Geometry: see drawing. Coordinates: mm, zero at the bounding-box minimum. Round coordinates to 2 decimals unless told otherwise and drop trailing zeros. Write each loop counter-clockwise with the first axis right and the second up, starting at its lowest first coordinate (ties: lowest second). Pieces come first, ordered by that corner, then holes. Notation, with made-up numbers: (7.5, 37.5) - (11.5, 37.5) arc R17 ccw to (11.5, 56.5) - close; hole circle Ø1 at (77, 76.25). An arc over 180 degrees is marked (long way). One line per item, written item: value. Start each with the question number.
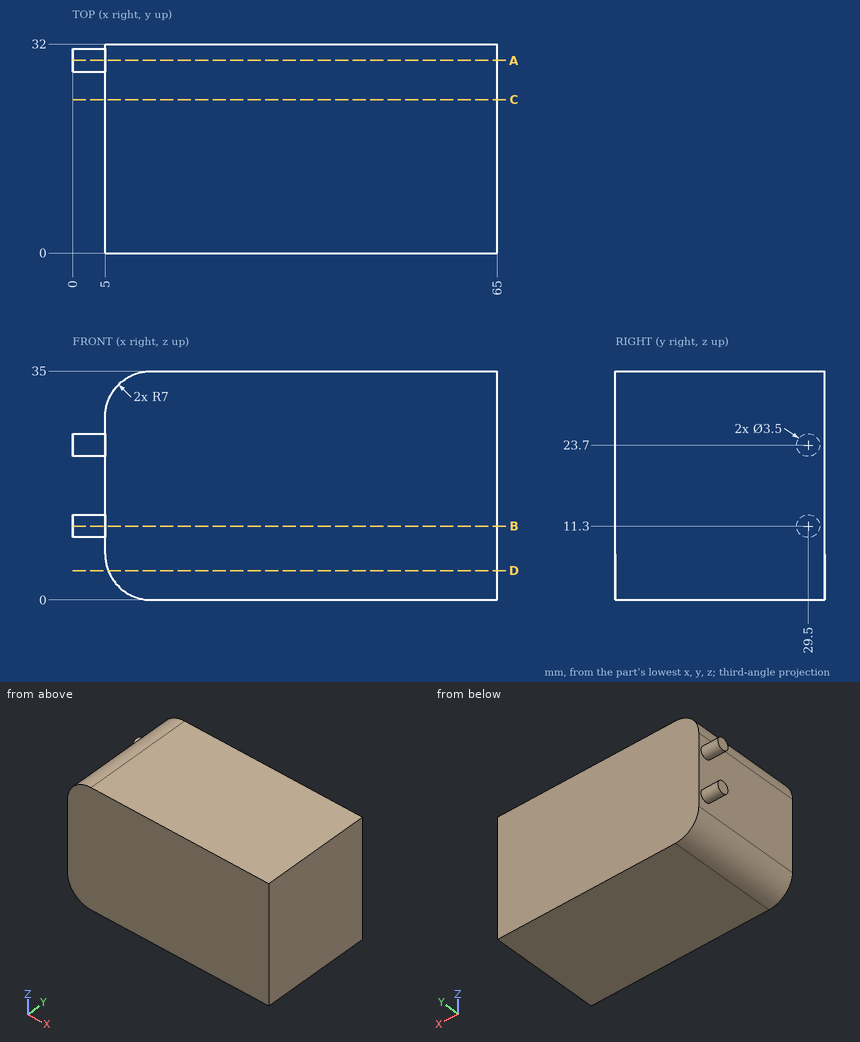
Q1. Material intervals for probe 1 along X at (y, z) = (30, 9); probe 2 along X at (y, z) = (9, 6); probe 3 along Z at (x, y) = (9, 18), sorted ascending. Write a range as from..to.
Q2. Cut plane B-B, the plane z = 11.3. Output: boundary loops of the cut face in (x, y), and give its area (3 significant figures).
Q3. Cut plane C-C, the plane y = 23.5. Output: boundary loops of the cut face in (x, z).
Q4. Cut plane A-A, the plane y = 29.5. Output: boundary loops of the cut face in (x, z).
Q5. Contact query for flat-ended pins moving along their axis: pin 1 Ø1 at (y, z) = (8.5, 5) entering from -X; pin 2 Ø6.5 at (y, z) = (21, 20.5) entering from -X. Output: stop coordinate, or through.
Q6. Cut plane D-D, the plane z = 4.5. Output: boundary loops of the cut face in (x, y), and give its area (3 significant figures).
A:
1. probe 1: x = 5..65
1. probe 2: x = 5.07..65
1. probe 3: z = 0.68..34.32
2. outline: (0, 27.75) - (5, 27.75) - (5, 0) - (65, 0) - (65, 32) - (5, 32) - (5, 31.25) - (0, 31.25) - close
2. area: 1,940 mm²
3. outline: (5, 7) arc R7 ccw to (12, 0) - (65, 0) - (65, 35) - (12, 35) arc R7 ccw to (5, 28) - close
4. outline: (0, 9.55) - (5, 9.55) - (5, 7) arc R7 ccw to (12, 0) - (65, 0) - (65, 35) - (12, 35) arc R7 ccw to (5, 28) - (5, 25.45) - (0, 25.45) - (0, 21.95) - (5, 21.95) - (5, 13.05) - (0, 13.05) - close
5. pin 1: stops at x = 5.16
5. pin 2: stops at x = 5
6. outline: (5.46, 0) - (65, 0) - (65, 32) - (5.46, 32) - close
6. area: 1,910 mm²
